For this review, take the finished solid that the model builds, in its own axes (mm). A direction names the side the tool comes from. Round coordinates to 2 decimals unless told otherwise and drop trailing zeros. Order: outer loops, then holes, each group sorted by start corner. A loop starts at its lowest first (then second) coordinate and runs counter-clockwise, first axis right, second up. Notation, with made-up numbers: (88.5, 57) -> (119.5, 57) arc R15 cw to (119.5, 70) -> close; hole circle Ø6 at (62.25, -32.5). An arc over 180 degrees is marked (long way). Use a Markdown table: item, result. Add a question column.
1) Consider section A-A (x = -42.5). State the section outline as (y, z) points, plus the area to 3 significant figures.
2) Clearance check with flat-ended pins moving along their axes: P1, Ø2, axis at x = -35, y = 9.5, coming from the +Z side; P2, Ø1.1, axis at y = 18.5, z = 6, coming from the +X side; P3, Ø2, axis at x = -37, y = -19.5, coming from the +Z side; P4, Ø5, axis at x = -17.5, y = 4, coming from the +Z side. State where each tip first meets the part, or that it passes through.
3) Wall thickness on line 1 along X through (y, z) = (8, -0.25); line 2 along Y through (x, z) = (-3.5, 0.75); line 3 along Y through (x, z) = (24.5, 2.75): over which ranges is each line inside the solid? List them lowest first. Write a range as [from, to].
4) Consider section C-C (z = 4). Give the number of separate pieces and of enclosed holes in the cut face, plus the area to 3 significant figures.
5) Machinability: for faces 4 (the face through (51.2, 8.8, 1.078)), 5 (the face through (-45.087, 19, 5)), 6 (the face through (10, -18.25, 0)), which of the approach directions +Z, -Z, +X, -X, +Y, -Y give a long, thin tool a straight path to every point of the face, cutting with its end or side? Answer none if there is none.
6) Consider section B-B (y = 0). State the section outline as (x, z) points.
7) Draft analysis for pull direction X (two halves, no side actions). For faces 1 (the face through (46, 0, 3)), 2 (the face through (52, 0, 3)), 3 (the face through (51.2, -9, 1.078)), state which applies: pulls with the +X half, pulls with the -X half, needs draft (parallel to the pull), parting line crosses it, or undercut.
8) Consider section D-D (x = -4.5). State the section outline as (y, z) points.
```python
from build123d import *

# Parameters (mm, degrees)
SKETCH002_W          = 100
SKETCH002_H          = 36.5
PAD002_DEPTH         = 12
THICKNESS_T          = 2
POCKET_DEPTH         = 9.001
SKETCH018_W          = 11.43
SKETCH018_H          = 15.122581
POCKET001_DEPTH      = 52.001
SKETCH019_W          = 11.43
SKETCH019_H          = 14.044283
POCKET002_DEPTH      = 20.251
POCKET002_DEPTH_BACK = 20.251
SKETCH003_R          = 1
PAD003_DEPTH         = 5
FILLET_R             = 1.5


with BuildPart() as part:
    # Sketch002 → Pad002 (new body)
    with BuildSketch(Plane.XY):
        Rectangle(SKETCH002_W, SKETCH002_H)
    extrude(amount=PAD002_DEPTH)

    # Thickness
    thickness_openings = [part.faces().sort_by_distance(p)[0] for p in [
        (0, 0, 12),
    ]]
    offset(amount=THICKNESS_T, openings=thickness_openings)

    # Sketch012 → Pocket (cut, through all)
    with BuildSketch(Plane.XY.offset(3)):
        Polygon((-25, 19.25), (25, 19.25), (25, 9.125), (51, 9.125), (51, -9.125), (25, -9.125), (25, -19.25), (-25, -19.25), (-25, -9.125), (-51, -9.125), (-51, 9.125), (-25, 9.125), align=None)
    extrude(amount=POCKET_DEPTH, mode=Mode.SUBTRACT)

    # Sketch018 → Pocket001 (cut, through all)
    with BuildSketch(Plane.YZ):
        with Locations((-7.62, 10.638799)):
            Rectangle(SKETCH018_W, SKETCH018_H)
        with Locations((7.62, 10.638799)):
            Rectangle(SKETCH018_W, SKETCH018_H)
    extrude(amount=POCKET001_DEPTH, mode=Mode.SUBTRACT)

    # Sketch019 → Pocket002 (cut, two sides)
    with BuildSketch(Plane.XZ) as pocket002_sk:
        with Locations((-39.372, 10.143712)):
            Rectangle(SKETCH019_W, SKETCH019_H)
    extrude(amount=POCKET002_DEPTH, mode=Mode.SUBTRACT)
    extrude(pocket002_sk.sketch, amount=-POCKET002_DEPTH_BACK, mode=Mode.SUBTRACT)

    # Sketch003 → Pad003 (join)
    with BuildSketch(Plane.XY):
        with Locations((-35.562, 9.526)):
            Circle(SKETCH003_R)
        with Locations((45.722, 0)):
            Circle(SKETCH003_R)
    extrude(amount=PAD003_DEPTH)

    # Fillet
    fillet_edges = [part.edges().sort_by_distance(p)[0] for p in [
        (0, 18.25, 0),
        (-50, 0, 0),
        (50, 0, 0),
        (0, -18.25, 0),
        (44.722, 0, 0),
        (-36.562, 9.526, 0),
    ]]
    fillet(fillet_edges, radius=FILLET_R)


with BuildPart() as part_1:
    # Body001 placement: moved
    add(part.part.moved(Location((0, 0, -2))))


solid = part_1.part
```
Results list:
| question | item | result |
|---|---|---|
| 1 | outline | (-20.25, -2) arc R2 ccw to (-18.25, -4) -> (18.25, -4) arc R2 ccw to (20.25, -2) -> (20.25, 1.12) -> (18.25, 1.12) -> (18.25, -0.5) arc R1.5 cw to (16.75, -2) -> (-16.75, -2) arc R1.5 cw to (-18.25, -0.5) -> (-18.25, 1.12) -> (-20.25, 1.12) -> close |
| 1 | area | 92.7 mm2 |
| 2 | P1 | z = 3 |
| 2 | P2 | x = 52 |
| 2 | P3 | z = 1.12 |
| 2 | P4 | z = -2 |
| 3 | line 1 | [-52, -50], [50, 52] |
| 3 | line 2 | [-20.25, -18.25], [18.25, 20.25] |
| 3 | line 3 | [-20.25, -19.25], [19.25, 20.25] |
| 4 | separate pieces | 4 |
| 4 | enclosed holes | 0 |
| 4 | area | 345 mm2 |
| 5 | face 4 | +Z, +X |
| 5 | face 5 | +Z, +Y, -Y |
| 5 | face 6 | +Z |
| 6 | outline | (-52, -2) arc R2 ccw to (-50, -4) -> (50, -4) arc R2 ccw to (52, -2) -> (52, 10) -> (51, 10) -> (51, 1) -> (50, 1) -> (50, -0.5) arc R1.5 cw to (48.5, -2) -> (48.22, -2) arc R1.5 cw to (46.72, -0.5) -> (46.72, 3) -> (44.72, 3) -> (44.72, -0.5) arc R1.5 cw to (43.22, -2) -> (-48.5, -2) arc R1.5 cw to (-50, -0.5) -> (-50, 1) -> (-51, 1) -> (-51, 10) -> (-52, 10) -> close |
| 7 | face 1 | undercut |
| 7 | face 2 | pulls with the +X half |
| 7 | face 3 | needs draft |
| 8 | outline | (-20.25, -2) arc R2 ccw to (-18.25, -4) -> (18.25, -4) arc R2 ccw to (20.25, -2) -> (20.25, 10) -> (19.25, 10) -> (19.25, 1) -> (18.25, 1) -> (18.25, -0.5) arc R1.5 cw to (16.75, -2) -> (-16.75, -2) arc R1.5 cw to (-18.25, -0.5) -> (-18.25, 1) -> (-19.25, 1) -> (-19.25, 10) -> (-20.25, 10) -> close |
